Work out the finished part from the listing and answer in its coordinate system (mm). Coordinates: 2 decimals unless noted, no trailing zeros. Write each loop counter-clockwise with the first axis right and the second up, starting at its lowest first coordinate (ties: lowest second). Pieces come first, ordered by that corner, then holes. Notation, with made-up numbers: (13.25, 44.5) - (45.25, 44.5) arc R11 ccw to (45.25, 65.5) - close; hole circle Ø11 at (52, -23). An arc over 180 degrees is marked (long way). One line per item, written item: value.
```python
from build123d import *

# Parameters (mm, degrees)
SKETCH_1_R           = 1
EXTRUDE_1_DEPTH      = 2
SKETCH_2_R           = 1
EXTRUDE_2_DEPTH      = 2
EXTRUDE_2_DEPTH_BACK = 4


with BuildPart() as part:
    # 草图1 → 凸台-拉伸1 (new body)
    with BuildSketch(Plane.XY):
        with BuildLine():
            Line((-50.159162871, -2), (99.840837129, -2))
            ThreePointArc((99.840837129, -2), (101.840837129, 0), (99.840837129, 2))
            Line((99.840837129, 2), (-50.159162871, 2))
            ThreePointArc((-50.159162871, 2), (-52.159162871, 0), (-50.159162871, -2))
        make_face()
        with Locations((99.840837129, 0)):
            Circle(SKETCH_1_R, mode=Mode.SUBTRACT)
    extrude(amount=EXTRUDE_1_DEPTH)

    # 草图2 → 凸台-拉伸2 (add, two sides)
    with BuildSketch(Plane.XY.offset(2)) as extrude_2_sk:
        with Locations((-50.159162871, 0)):
            Circle(SKETCH_2_R)
    extrude(amount=EXTRUDE_2_DEPTH)
    extrude(extrude_2_sk.sketch, amount=-EXTRUDE_2_DEPTH_BACK)


solid = part.part
```
Item 1: Section B-B, the plane x = 88 is taken. Determine the outline of the cut face in (y, z).
Evaluation:
outline: (-2, 0) - (2, 0) - (2, 2) - (-2, 2) - close
Item 2: Section A-A, the plane y = 0 is taken. Determine the outline of the cut face in (x, z).
Evaluation:
outline: (-52.16, 0) - (-51.16, 0) - (-51.16, -2) - (-49.16, -2) - (-49.16, 0) - (98.84, 0) - (98.84, 2) - (-49.16, 2) - (-49.16, 4) - (-51.16, 4) - (-51.16, 2) - (-52.16, 2) - close; (100.84, 0) - (101.84, 0) - (101.84, 2) - (100.84, 2) - close
Item 3: Consider probe 1 along Z at (x, y) = (4, -1.3); probe 2 along X at (y, z) = (0.6, 1.2); probe 3 along X at (y, z) = (0.4, -0.55). Determine where each line is inside the solid, lowest interval first.
Evaluation:
probe 1: z = 0 to 2
probe 2: x = -52.07 to 99.04, 100.64 to 101.75
probe 3: x = -51.08 to -49.24
Item 4: Given pin 1 (1.6 mm diameter, centred on x = 99.84, y = 0, fed in from +Z); pin 2 (1.2 mm diameter, centred on x = 7, y = 0.5, fed in from -Z), each flat-ended and moving along its own axis, determine where each tip first touches the part or whether it passes through.
Evaluation:
pin 1: passes through
pin 2: stops at z = 0
